Geometry: final body of the model. Coordinates: model frame, mm. Give positions to 0.01 mm unless a question says otherwise; leave off trailing zeros. Loops run counter-clockwise (first coordinate to the right, second up) from the corner with the lowest first, then second, coordinate; pieces in that order, holes last. Notation, with made-up numbers: (2, 85.5) - (52, 85.5) arc R26 ccw to (52, 103.5) - close; hole circle Ø1 at (32.25, 60). An arc over 180 degrees is marked (long way). Use CSV: the item, a comma, the result in double quotes. Start each with the question number.
```python
from build123d import *

# Parameters (mm, degrees)
IZIM2_R                     = 1.6
Y_KSEKLIK_EKSTR_ZYON1_DEPTH = 2
IZIM3_R                     = 2.25
KES_EKSTR_ZYON1_DEPTH       = 2


with BuildPart() as part:
    # Çizim2 → Yükseklik-Ekstrüzyon1 (new body)
    with BuildSketch(Plane.YZ):
        with BuildLine():
            Line((-77.099299539, -127.848423963), (-64.349299539, -127.848423963))
            Line((-64.349299539, -127.848423963), (-64.349299539, -130.848423963))
            ThreePointArc((-64.349299539, -130.848423963), (-60.599299539, -134.598423963), (-56.849299539, -130.848423963))
            Line((-56.849299539, -130.848423963), (-56.849299539, -127.848423963))
            Line((-56.849299539, -127.848423963), (55.650700461, -127.848423963))
            Line((55.650700461, -127.848423963), (55.650700461, -130.848423963))
            ThreePointArc((55.650700461, -130.848423963), (59.400700461, -134.598423963), (63.150700461, -130.848423963))
            Line((63.150700461, -130.848423963), (63.150700461, -127.848423963))
            Line((63.150700461, -127.848423963), (75.900700461, -127.848423963))
            ThreePointArc((75.900700461, -127.848423963), (79.436234367, -126.383957869), (80.900700461, -122.848423963))
            Line((80.900700461, -122.848423963), (80.900700461, -80.764464123))
            Line((80.900700461, -80.764464123), (83.900700461, -80.764464123))
            ThreePointArc((83.900700461, -80.764464123), (87.650700461, -77.014464123), (83.900700461, -73.264464123))
            Line((83.900700461, -73.264464123), (80.900700461, -73.264464123))
            Line((80.900700461, -73.264464123), (80.900700461, -0.764464123))
            Line((80.900700461, -0.764464123), (83.900700461, -0.764464123))
            ThreePointArc((83.900700461, -0.764464123), (87.650700461, 2.985535877), (83.900700461, 6.735535877))
            Line((83.900700461, 6.735535877), (80.900700461, 6.735535877))
            Line((80.900700461, 6.735535877), (80.900700461, 79.235535877))
            Line((80.900700461, 79.235535877), (83.900700461, 79.235535877))
            ThreePointArc((83.900700461, 79.235535877), (87.650700461, 82.985535877), (83.900700461, 86.735535877))
            Line((83.900700461, 86.735535877), (80.900700461, 86.735535877))
            Line((80.900700461, 86.735535877), (80.900700461, 120.151576037))
            ThreePointArc((80.900700461, 120.151576037), (79.436234367, 123.687109943), (75.900700461, 125.151576037))
            Line((75.900700461, 125.151576037), (63.150700461, 125.151576037))
            Line((63.150700461, 125.151576037), (63.150700461, 128.151576037))
            ThreePointArc((63.150700461, 128.151576037), (59.400700461, 131.901576037), (55.650700461, 128.151576037))
            Line((55.650700461, 128.151576037), (55.650700461, 125.151576037))
            Line((55.650700461, 125.151576037), (-56.849299539, 125.151576037))
            Line((-56.849299539, 125.151576037), (-56.849299539, 128.151576037))
            ThreePointArc((-56.849299539, 128.151576037), (-60.599299539, 131.901576037), (-64.349299539, 128.151576037))
            Line((-64.349299539, 128.151576037), (-64.349299539, 125.151576037))
            Line((-64.349299539, 125.151576037), (-77.099299539, 125.151576037))
            ThreePointArc((-77.099299539, 125.151576037), (-80.634833445, 123.687109943), (-82.099299539, 120.151576037))
            Line((-82.099299539, 120.151576037), (-82.099299539, 86.735535877))
            Line((-82.099299539, 86.735535877), (-85.099299539, 86.735535877))
            ThreePointArc((-85.099299539, 86.735535877), (-88.849299539, 82.985535877), (-85.099299539, 79.235535877))
            Line((-85.099299539, 79.235535877), (-82.099299539, 79.235535877))
            Line((-82.099299539, 79.235535877), (-82.099299539, 6.735535877))
            Line((-82.099299539, 6.735535877), (-85.099299539, 6.735535877))
            ThreePointArc((-85.099299539, 6.735535877), (-88.849299539, 2.985535877), (-85.099299539, -0.764464123))
            Line((-85.099299539, -0.764464123), (-82.099299539, -0.764464123))
            Line((-82.099299539, -0.764464123), (-82.099299539, -73.264464123))
            Line((-82.099299539, -73.264464123), (-85.099299539, -73.264464123))
            ThreePointArc((-85.099299539, -73.264464123), (-88.849299539, -77.014464123), (-85.099299539, -80.764464123))
            Line((-85.099299539, -80.764464123), (-82.099299539, -80.764464123))
            Line((-82.099299539, -80.764464123), (-82.099299539, -122.848423963))
            ThreePointArc((-82.099299539, -122.848423963), (-80.634833445, -126.383957869), (-77.099299539, -127.848423963))
        make_face()
        with Locations(Location((-85.099299539, 82.985535877, 0), (0, 0, 270))):
            Circle(IZIM2_R, mode=Mode.SUBTRACT)
        with Locations(Location((-85.099299539, 2.985535877, 0), (0, 0, 270))):
            Circle(IZIM2_R, mode=Mode.SUBTRACT)
        with Locations(Location((-85.099299539, -77.014464123, 0), (0, 0, 270))):
            Circle(IZIM2_R, mode=Mode.SUBTRACT)
        with Locations(Location((-60.599299539, -130.848423963, 0), (0, 0, 270))):
            Circle(IZIM2_R, mode=Mode.SUBTRACT)
        with Locations(Location((59.400700461, -130.848423963, 0), (0, 0, 270))):
            Circle(IZIM2_R, mode=Mode.SUBTRACT)
        with Locations(Location((83.900700461, -77.014464123, 0), (0, 0, 270))):
            Circle(IZIM2_R, mode=Mode.SUBTRACT)
        with Locations(Location((83.900700461, 2.985535877, 0), (0, 0, 270))):
            Circle(IZIM2_R, mode=Mode.SUBTRACT)
        with Locations(Location((83.900700461, 82.985535877, 0), (0, 0, 270))):
            Circle(IZIM2_R, mode=Mode.SUBTRACT)
        with Locations(Location((59.400700461, 128.151576037, 0), (0, 0, 270))):
            Circle(IZIM2_R, mode=Mode.SUBTRACT)
        with Locations(Location((-60.599299539, 128.151576037, 0), (0, 0, 270))):
            Circle(IZIM2_R, mode=Mode.SUBTRACT)
    extrude(amount=Y_KSEKLIK_EKSTR_ZYON1_DEPTH)

    # Çizim3 → Kes-Ekstrüzyon1 (cut)
    with BuildSketch(Plane.YZ.offset(2)):
        with Locations(Location((-60.599299539, 128.151576037, 0), (0, 0, 270))):
            Circle(IZIM3_R)
    kes_ekstr_zyon1 = extrude(amount=-KES_EKSTR_ZYON1_DEPTH, mode=Mode.SUBTRACT)

    # Çizim-Çoğaltma1: Kes-Ekstrüzyon1 at 10 more places
    with Locations((0, 120, 0), (0, 144.5, -45.16604), (0, 144.5, -125.16604), (0, 144.5, -205.16604), (0, 120, -259), (0, 0, -259), (0, -24.5, -205.16604), (0, -24.5, -125.16604), (0, -24.5, -45.16604), (0, -147.335631, 64.588173)):
        add(kes_ekstr_zyon1, mode=Mode.SUBTRACT)


solid = part.part
```
Item 1: Section A-A (z = -22). Output: boundary loops of the cut face in (x, y).
Item 2: Section C-C (x = 0.3). Give the number of separate pieces and of enclosed holes in the cut face, plus the area to 3 significant figures.
Item 3: Section B-B (y = 0.5). Output: boundary loops of the cut face in (x, z), plus the area to 3 significant figures.
Item 4: Ray query, probe 1 along Z at (x, y) = (0.25, 49); probe 2 along Y at (x, z) = (1, 66.5); probe 3 along Y at (x, z) = (1.15, -74.5). Return the intervals inside material, ascending.
Item 5: Mould query, pull axis X, two halves, no side actions, for faces 1 (the cylindrical face through (0.99, 79.4, -126.42)), 2 (the flat face through (2, -2, 1)), 3 (the flat face through (0, -2, 1)). Classes: pulls with the +X half, pulls with the -X half, needs draft (parallel to the pull), parting line crosses it, or undercut.
Item 6: Pin query (flat end, axial travel): pin 1 Ø1 at (x, z) = (0.5, 41) entering from -Y; pin 2 Ø1 at (x, z) = (1.5, 55.5) entering from +Y; pin 3 Ø1 at (x, y) = (1, 14) entering from +Z. Return the tip coordinate at first contact, or that it passes through.
Outcome:
1,outline,"(0, -82.1) - (2, -82.1) - (2, 80.9) - (0, 80.9) - close"
2,separate pieces,"1"
2,enclosed holes,"10"
2,area,"41,500 mm2"
3,outline,"(0, -127.85) - (2, -127.85) - (2, 125.15) - (0, 125.15) - close"
3,area,"506 mm2"
4,probe 1,"z = -127.85 to 125.15"
4,probe 2,"y = -82.1 to 80.9"
4,probe 3,"y = -87.88 to 86.68"
5,face 1,"needs draft"
5,face 2,"pulls with the +X half"
5,face 3,"pulls with the -X half"
6,pin 1,"stops at y = -82.1"
6,pin 2,"stops at y = 80.9"
6,pin 3,"stops at z = 125.15"
